Autodesk Inventor part; units mm, degrees
ref_plane "Work Plane2" through (0, -62, -224) normal (1, 0, 0) x (0, 0, -1)
ref_plane "YZ Plane" through (0, 0, 0) normal (1, 0, 0) x (0, 1, 0)
ref_plane "XZ Plane" through (0, 0, 0) normal (0, 1, 0) x (-1, 0, 0)
sketch "Sketch1" plane through (0, 0, 0) normal (0, 1, 0) x (-1, 0, 0)
  line L0 (-152.5, -224) -> (152.5, -224)
  line L1 (152.5, -224) -> (152.5, 224)
  line L2 (152.5, 224) -> (-152.5, 224)
  line L3 (-152.5, 224) -> (-152.5, -224)
  line L4 (-152.5, -224) -> (152.5, 224) construction
  line L5 (152.5, -224) -> (-152.5, 224) construction
  point P0 (0, 0)
  point P1 (132, 210)
  point P2 (-132, -210)
  point P3 (132, -210)
  point P4 (-132, 210)
  dimension "d0" = 305
  dimension "d1" = 448
extrude "Extrusion1" add sketch "Sketch1" along normal blind 3
sketch "Sketch2" plane through (0, 3, 0) normal (0, 1, 0) x (1, 0, 0)
  line L0 (-152.5, 224) -> (-152.5, -224)
  line L1 (-152.5, -224) -> (152.5, -224)
  line L2 (152.5, -224) -> (152.5, 224)
  line L3 (152.5, 224) -> (-152.5, 224)
  line L4 (-152.5, 224) -> (-152.5, -224)
  line L5 (-152.5, -224) -> (152.5, -224)
  line L6 (152.5, -224) -> (152.5, 224)
  line L7 (152.5, 224) -> (-152.5, 224)
  line L8 (-149.5, -221) -> (-149.5, 221)
  line L9 (-149.5, 221) -> (149.5, 221)
  line L10 (149.5, 221) -> (149.5, -221)
  line L11 (149.5, -221) -> (-149.5, -221)
  point P0 (0, 0)
  dimension "d4" = 3
extrude "Extrusion2" add sketch "Sketch2" along normal blind 50 and the other way blind 65
hole "Hole1" at (132, 0, -210) at (132, 0, 210) at (-132, 0, 210) at (-132, 0, -210) direction (0, 1, 0) diameter 5 end through all
sketch "Sketch3" plane through (152.5, -62, -224) normal (1, 0, 0) x (0, 0, -1)
  line L0 (0, 0) -> (0, 115)
  line L1 (-448, 115) -> (0, 115)
  line L2 (-448, 0) -> (-448, 115)
  line L3 (0, 0) -> (-448, 0)
  point P0 (-224, 62)
sketch "Sketch4" plane through (152.5, -62, -224) normal (1, 0, 0) x (0, 0, -1)
  line L0 (0, 0) -> (0, 115)
  line L1 (-448, 115) -> (0, 115)
  line L2 (-448, 0) -> (-448, 115)
  line L3 (0, 0) -> (-448, 0)
  point P0 (-224, 62)
sketch "Sketch5" plane through (152.5, -62, -224) normal (1, 0, 0) x (0, 0, -1)
  line L0 (0, 0) -> (0, 115)
  line L1 (-448, 115) -> (0, 115)
  line L2 (-448, 0) -> (-448, 115)
  line L3 (0, 0) -> (-448, 0)
  line L4 (0, 0) -> (-448, 0)
  point P0 (-224, 62)
  point P1 (-224, 62)
  point P2 (-99, 25)
  dimension "d16" = 99
  dimension "d17" = 25
sketch "Sketch6" plane through (152.5, -62, -224) normal (1, 0, 0) x (0, 0, -1)
  line L0 (0, 0) -> (-448, 0)
  line L1 (-445, 115) -> (-3, 115)
  line L2 (-224, 115) -> (-224, 0)
  line L3 (-78, 0) -> (-120, 0)
  line L4 (-120, 0) -> (-120, 30)
  line L5 (-100, 50) -> (-98, 50)
  line L6 (-78, 30) -> (-78, 0)
  line L7 (-78, 0) -> (-120, 50) construction
  line L8 (-120, 0) -> (-78, 50) construction
  line L9 (-448, 0) -> (-448, 115)
  arc A0 (-100, 50) -> (-120, 30) centre (-100, 30) ccw
  arc A1 (-78, 30) -> (-98, 50) centre (-98, 30) ccw
  line L10 (-328, 0) -> (-328, 30)
  line L11 (-370, 30) -> (-370, 0)
  line L12 (-370, 0) -> (-328, 50) construction
  line L13 (-328, 0) -> (-370, 50) construction
  arc A2 (-328, 30) -> (-348, 50) centre (-348, 30) ccw
  arc A3 (-350, 50) -> (-370, 30) centre (-350, 30) ccw
  line L14 (-304.3108, 54.0001) -> (-144.3108, 54.0001) construction
  line L15 (-445, 62) -> (-3, 62)
  line L16 (-304.3108, 36.5001) -> (-144.3108, 36.5001)
  line L17 (-144.3108, 71.5001) -> (-304.3108, 71.5001)
  arc A4 (-304.3108, 71.5001) -> (-304.3108, 36.5001) centre (-304.3108, 54.0001) ccw
  arc A5 (-144.3108, 36.5001) -> (-144.3108, 71.5001) centre (-144.3108, 54.0001) ccw
  line L18 (-370, 0) -> (-328, 0)
  line L19 (-328, 0) -> (-328, 30)
  line L20 (-328, 30) -> (-370, 30)
  line L21 (-370, 30) -> (-370, 0)
  line L22 (-350, 50) -> (-348, 50)
  point P0 (-224, 62)
  point P1 (-99, 25)
  point P2 (-99, 25)
  point P3 (-99, 25)
  point P4 (-120, 0)
  point P5 (-78, 0)
  point P6 (-349, 25)
  point P7 (-349, 25)
  point P8 (-99, 50)
  point P9 (-349, 50)
  point P10 (-370, 0)
  point P11 (-328, 0)
  point P12 (-224.3108, 54.0001)
  point P13 (-304.3108, 54.0001)
  dimension "d18" = 42
  dimension "d19" = 50
  dimension "d26" = 20
  dimension "d27" = 20
  dimension "d28" = 99
  dimension "d29" = 25
  dimension "d32" = 35
extrude "Extrusion3" cut sketch "Sketch6" against normal through all contours L0 L4 A0 L5 A1 L6
extrude "Extrusion4" cut sketch "Sketch6" against normal through all contours L0 L11 L20 L10 | L20 A3 L22 A2
extrude "Extrusion5" cut sketch "Sketch6" against normal blind 3 contours L16 A4 L15 L2 | L2 L15 A5 L16 | L15 A4 L17 L2 | L2 L17 A5 L15
sketch "Sketch7" plane through (152.5, -62, -224) normal (1, 0, 0) x (0, 0, -1)
  arc A0 (-144.3108, 36.5001) -> (-144.3108, 71.5001) centre (-144.3108, 54.0001) ccw
  line L0 (-144.3108, 36.5001) -> (-304.3108, 36.5001)
  arc A1 (-304.3108, 71.5001) -> (-304.3108, 36.5001) centre (-304.3108, 54.0001) ccw
  line L1 (-304.3108, 71.5001) -> (-144.3108, 71.5001)
  line L2 (-370, 0) -> (-370, 30)
  arc A2 (-328, 30) -> (-348, 50) centre (-348, 30) ccw
  line L3 (-328, 30) -> (-328, 0)
  line L4 (-120, 0) -> (-328, 0)
  line L5 (-120, 0) -> (-120, 30)
  arc A3 (-100, 50) -> (-120, 30) centre (-100, 30) ccw
  line L6 (-78, 30) -> (-78, 0)
  line L7 (0, 0) -> (-78, 0)
  line L8 (0, 0) -> (0, 115)
  line L9 (-448, 115) -> (0, 115)
  line L10 (-448, 0) -> (-448, 115)
  line L11 (-370, 0) -> (-448, 0)
  point P0 (-369, 30)
  point P1 (-79, 30)
  point P2 (-224, 62)
ref_plane "Work Plane2" through (0, -62, -224) normal (1, 0, 0) x (0, 0, -1)
sketch "Sketch8" plane through (152.5, -62, -224) normal (1, 0, 0) x (0, 0, -1)
  arc A0 (-144.3108, 36.5001) -> (-144.3108, 71.5001) centre (-144.3108, 54.0001) ccw
  line L0 (-144.3108, 36.5001) -> (-304.3108, 36.5001)
  arc A1 (-304.3108, 71.5001) -> (-304.3108, 36.5001) centre (-304.3108, 54.0001) ccw
  line L1 (-304.3108, 71.5001) -> (-144.3108, 71.5001)
  line L2 (-370, 0) -> (-370, 30)
  arc A2 (-328, 30) -> (-348, 50) centre (-348, 30) ccw
  line L3 (-328, 30) -> (-328, 0)
  line L4 (-120, 0) -> (-328, 0)
  line L5 (-120, 0) -> (-120, 30)
  arc A3 (-100, 50) -> (-120, 30) centre (-100, 30) ccw
  line L6 (-78, 30) -> (-78, 0)
  line L7 (0, 0) -> (-78, 0)
  line L8 (0, 0) -> (0, 115)
  line L9 (-448, 115) -> (0, 115)
  line L10 (-448, 0) -> (-448, 115)
  line L11 (-370, 0) -> (-448, 0)
  point P0 (-369, 30)
  point P1 (-79, 30)
  point P2 (-224, 62)
mirror "Mirror1" about plane through (0, -62, -224) normal (1, 0, 0) of "Extrusion5"
properties part number "AMR_Top_Basket" material "Aluminum 6061"
Could you check a few things on this model? Use its own coordinates, in mm. A direction names the side the tool comes from. Coordinates: 2 decimals unless noted, no trailing zeros. Write each loop counter-clockwise with the first axis right and the second up, starting at its lowest first coordinate (ties: lowest second). Pieces come first, ordered by that corner, then holes. Notation, with made-up numbers: M -20.75,72 L -7.75,72 A10 ccw -7.75,86 Z; hole C 22.5,86 d6. An arc over 180 degrees is marked long. One line per question, with ' | ' between items.
1) Imagine slicing it at C-C, the plane z = -177. Write out the boundary of the cut face in (x, y).
Checks:
outline: M -152.5,-62 L -149.5,-62 L -149.5,0 L 149.5,0 L 149.5,-62 L 152.5,-62 L 152.5,53 L 149.5,53 L 149.5,3 L -149.5,3 L -149.5,53 L -152.5,53 Z
2) Imagine slicing it at A-A, the plane y = -48. Write out the boundary of the cut face in (x, z), and give its area (3 significant figures).
Checks:
outline: M -152.5,-224 L 152.5,-224 L 152.5,-146 L 149.5,-146 L 149.5,-221 L -149.5,-221 L -149.5,-146 L -152.5,-146 Z; M -152.5,-104 L -149.5,-104 L -149.5,104 L -152.5,104 Z; M -152.5,146 L -149.5,146 L -149.5,221 L 149.5,221 L 149.5,146 L 152.5,146 L 152.5,224 L -152.5,224 Z; M 149.5,-104 L 152.5,-104 L 152.5,104 L 149.5,104 Z | area: 3,980 mm²
3) For faces 1 (the face through (-150.979, -17.703, -110.014)), 2 (the face through (-2, -5, 224)), 3 (the face through (-149.5, 28, 3)), 4 (the face through (-2, -31, -221)), 5 (the face through (-1, -62, -223)), which set-ups out of +Z, -Z, +X, -X, +Y, -Y let a thin tool reach every point of the face, with its end or its side?
Checks:
face 1: +X, -X, -Y | face 2: +Z, +X, -X, +Y, -Y | face 3: +Y | face 4: -Y | face 5: +Z, -Z, +X, -X, -Y
4) Imagine slicing it at B-B, the plane z = -38. Write out the boundary of the cut face in (x, y), and give its area (3 significant figures).
Checks:
outline: M -152.5,-62 L -149.5,-62 L -149.5,-25.5 L -152.5,-25.5 Z; M -152.5,9.5 L -149.5,9.5 L -149.5,53 L -152.5,53 Z; M -149.5,0 L 149.5,0 L 149.5,3 L -149.5,3 Z; M 149.5,-62 L 152.5,-62 L 152.5,-25.5 L 149.5,-25.5 Z; M 149.5,9.5 L 152.5,9.5 L 152.5,53 L 149.5,53 Z | area: 1,380 mm²
5) Imagine slicing it at D-D, the plane y = 14. Write out the boundary of the cut face in (x, z).
Checks:
outline: M -152.5,-224 L 152.5,-224 L 152.5,224 L -152.5,224 Z; hole M -149.5,-221 L 149.5,-221 L 149.5,221 L -149.5,221 Z
6) I need wall thicknesses on probe 1 along X at (y, z) = (1.1, -210); probe 2 along Z at (x, y) = (132, 1.35); probe 3 along Z at (x, y) = (-7, -40). Which ranges of each line are inside material? Lowest first, please. Write a range as [from, to].
Checks:
probe 1: [-152.5, -134.5], [-129.5, 129.5], [134.5, 152.5] | probe 2: [-224, -212.5], [-207.5, 207.5], [212.5, 224] | probe 3: [-224, -221], [221, 224]
7) If we mould it in two halves opening along Y, with no side actions, what happens to faces 6 (the face through (2, -31, 221)), 7 (the face through (151.021, -7.615, 97.807)), 8 (the face through (151.021, -17.703, 139.986))? For each: released by +Y, released by -Y, zero draft, split by the parting line, or undercut.
Checks:
face 6: zero draft | face 7: undercut | face 8: released by -Y
8) For pin 1 Ø4.5 at (x, z) = (132, 210) entering from -Y; pin 2 Ø4 at (x, z) = (59.5, -31.5) entering from -Y; pin 3 Ø2 at (x, z) = (151.5, -125) entering from -Y; pin 4 Ø2 at (x, z) = (53.5, 133) entering from +Y, each with a flat end and sliding along its axis, tell me the tip position at first contact or that it passes through.
Checks:
pin 1: through | pin 2: y = 0 | pin 3: y = -12 | pin 4: y = 3
